```python
from build123d import *

# Parameters (mm, degrees)
F1_DEPTH = 12.7
F2_DEPTH = 25.4


with BuildPart() as f1:
    # F0 (on Front) → F1 (new body)
    with BuildSketch(Plane.XZ):
        Polygon((-30.429008, 25.641112), (-30.429008, -11.671882), (-53.379117, -11.671882), (-69.406818, -33.085297), (-69.406818, -64.011575), (-31.320526, -64.011575), (-15.292825, -42.598161), (-15.292825, -23.857851), (26.74457, -23.857851), (26.74457, -40.639478), (48.158187, -56.666891), (88.203151, -56.666891), (88.203151, -27.699199), (66.789736, -11.671497), (41.867928, -11.671497), (41.867928, 25.641497), (66.789822, 25.641497), (88.203439, 41.66891), (88.203439, 70.636506), (48.158778, 70.636506), (26.74588, 54.608069), (26.74588, 37.331953), (-15.291514, 37.331953), (-15.291514, 54.607823), (-36.70624, 70.636506), (-76.751118, 70.636506), (-76.751118, 41.668814), (-55.337703, 25.641112), align=None)
    extrude(amount=F1_DEPTH)

    # F0 (on Front) → F2 (join, symmetric)
    with BuildSketch(Plane.XZ):
        Polygon((15.074383, 49.003451), (-3.620017, 49.003451), (-3.620017, 60.450634), (-32.822015, 82.308003), (-88.422615, 82.308003), (-88.422615, 35.826003), (-59.221928, 13.969615), (-42.100506, 13.969615), (-42.100506, -0.000385), (-59.221928, -0.000385), (-81.078316, -29.201073), (-81.078316, -75.683073), (-25.477716, -75.683073), (-3.621328, -46.482385), (-3.621328, -35.529348), (15.073072, -35.529348), (15.073072, -46.482385), (44.274048, -68.338388), (99.874648, -68.338388), (99.874648, -21.856388), (70.673961, 0), (53.539425, 0), (53.539425, 13.97), (70.673961, 13.97), (99.874936, 35.826003), (99.874936, 82.308003), (44.274336, 82.308003), (15.074383, 60.450634), align=None)
        Polygon((-53.379117, -11.671882), (-30.429008, -11.671882), (-30.429008, 25.641112), (-55.337703, 25.641112), (-76.751118, 41.668814), (-76.751118, 70.636506), (-36.70624, 70.636506), (-15.291514, 54.607823), (-15.291514, 37.331953), (26.74588, 37.331953), (26.74588, 54.608069), (48.158778, 70.636506), (88.203439, 70.636506), (88.203439, 41.66891), (66.789822, 25.641497), (41.867928, 25.641497), (41.867928, -11.671497), (66.789736, -11.671497), (88.203151, -27.699199), (88.203151, -56.666891), (48.158187, -56.666891), (26.74457, -40.639478), (26.74457, -23.857851), (-15.292825, -23.857851), (-15.292825, -42.598161), (-31.320526, -64.011575), (-69.406818, -64.011575), (-69.406818, -33.085297), align=None, mode=Mode.SUBTRACT)
    extrude(amount=F2_DEPTH, both=True)


solid = f1.part
```
Source: CAD feature listing. Evaluate the final solid. Frame: model axes, mm. A direction names the side the tool comes from. Round coordinates to 2 decimals unless told otherwise and drop trailing zeros. Loops run counter-clockwise (first coordinate to the right, second up) from the corner with the lowest first, then second, coordinate; pieces in that order, holes last. Notation, with made-up numbers: M -22,60 L 25,60 A18 cw 25,78 Z; hole C -26,-34.75 d6. An arc over 180 degrees is marked long. Use a Markdown table: item, result. Add a question column.
1. Ray query, line 1 along Z through (x, y) = (-41, 13.5); line 2 along Z through (x, y) = (56.5, 7); line 3 along X through (y, z) = (-20.5, -39). Return the intervals inside material, ascending. Write a range as [from, to].
2. Cut plane A-A, the plane y = -5. Output: boundary loops of the cut face in (x, z), and give its area (4 significant figures).
3. Contact query for flat-ended pins moving along their axis: pin 1 (4 mm diameter, centred on y = -16.5, z = 12, fed in from -X); pin 2 (10 mm diameter, centred on x = -57.5, z = -49, fed in from -Y); pin 3 (10 mm diameter, centred on y = -19.5, z = -44, fed in from -X). Output: stop coordinate, or through.
4. Cut plane D-D, the plane z = 8. Output: boundary loops of the cut face in (x, y), and give its area (3 significant figures).
5. Cut plane B-B, the plane z = 52. Output: boundary loops of the cut face in (x, y).
6. Set-up query: faces 1 (the flat face through (5, 13, 37.332)), 2 (the flat face through (-74.027, -0.356, 25.051)), 3 (the flat face through (6, 0, 49.003)). Return all of +Z, -Z, +X, -X, +Y, -Y with unobstructed straight access to the full face (end or side cutting, diameter ignored); none if empty.
7. Pull-direction query (X, two-part tool) for faces 4 (the flat face through (4, 25.4, 40)), 5 (the flat face through (-88.423, 0, 59)), 6 (the flat face through (5, -12.7, 4)); classes: +X half, -X half, draft (parallel to the pull), parting line (faces both ways), or undercut.
8. Cut plane C-C, the plane x = -67. Output: boundary loops of the cut face in (y, z).
Solution:
| question | item | result |
|---|---|---|
| 1 | line 1 | z = [-75.68, -64.01], [-11.67, 25.64], [70.64, 82.31] |
| 1 | line 2 | z = [-68.34, -56.67], [-11.67, 0], [13.97, 25.64], [70.64, 82.31] |
| 1 | line 3 | x = [-81.08, -69.41], [-15.29, -3.62], [15.07, 26.74], [88.2, 99.87] |
| 2 | outline | M -88.42,35.83 L -59.22,13.97 L -42.1,13.97 L -42.1,0 L -59.22,0 L -81.08,-29.2 L -81.08,-75.68 L -25.48,-75.68 L -3.62,-46.48 L -3.62,-35.53 L 15.07,-35.53 L 15.07,-46.48 L 44.27,-68.34 L 99.87,-68.34 L 99.87,-21.86 L 70.67,0 L 53.54,0 L 53.54,13.97 L 70.67,13.97 L 99.87,35.83 L 99.87,82.31 L 44.27,82.31 L 15.07,60.45 L 15.07,49 L -3.62,49 L -3.62,60.45 L -32.82,82.31 L -88.42,82.31 Z |
| 2 | area | 23,350 mm2 |
| 3 | pin 1 | stops at x = -59.26 |
| 3 | pin 2 | stops at y = -12.7 |
| 3 | pin 3 | stops at x = -81.08 |
| 4 | outline | M -42.1,-25.4 L -30.43,-25.4 L -30.43,-12.7 L 41.87,-12.7 L 41.87,-25.4 L 53.54,-25.4 L 53.54,25.4 L 41.87,25.4 L 41.87,0 L -30.43,0 L -30.43,25.4 L -42.1,25.4 Z |
| 4 | area | 2,100 mm2 |
| 5 | outline | M -88.42,-25.4 L -76.75,-25.4 L -76.75,-12.7 L -15.29,-12.7 L -15.29,-25.4 L -3.62,-25.4 L -3.62,25.4 L -15.29,25.4 L -15.29,0 L -76.75,0 L -76.75,25.4 L -88.42,25.4 Z; M 15.07,-25.4 L 26.75,-25.4 L 26.75,-12.7 L 88.2,-12.7 L 88.2,-25.4 L 99.87,-25.4 L 99.87,25.4 L 88.2,25.4 L 88.2,0 L 26.75,0 L 26.75,25.4 L 15.07,25.4 Z |
| 6 | face 1 | +Y |
| 6 | face 2 | -X, +Y, -Y |
| 6 | face 3 | +Z, +Y, -Y |
| 7 | face 4 | draft |
| 7 | face 5 | -X half |
| 7 | face 6 | undercut |
| 8 | outline | M -25.4,-75.68 L 25.4,-75.68 L 25.4,-64.01 L 0,-64.01 L 0,-29.87 L 25.4,-29.87 L 25.4,-10.39 L -25.4,-10.39 L -25.4,-29.87 L -12.7,-29.87 L -12.7,-64.01 L -25.4,-64.01 Z; M -25.4,19.79 L 25.4,19.79 L 25.4,34.37 L 0,34.37 L 0,70.64 L 25.4,70.64 L 25.4,82.31 L -25.4,82.31 L -25.4,70.64 L -12.7,70.64 L -12.7,34.37 L -25.4,34.37 Z |
